Geometry: see drawing. Coordinates: mm, zero at the bounding-box minimum. A direction names the side the tool comes from. Give positions to 0.01 mm unless a question says otherwise; leave off trailing zeros. Write each loop counter-clockwise with the first axis right and the second up, starting at its lowest first coordinate (ties: lowest second). Pieces come first, ordered by that corner, then holes. Notation, with made-up numbers: (48.5, -25) -> (79.5, -25) arc R30 cw to (79.5, 9) -> close; hole circle Ø8 at (7.5, 77). An arc over 180 degrees is marked (long way). Use one line per item in the form item = value. Start each with the question number.
(1) Set-up query: the marked faces 3 and 4. Return all of +Z, -Z, +X, -X, +Y, -Y with unobstructed straight access to the full face (end or side cutting, diameter ignored); none if empty.
(2) Material intervals for line 1 along X through (y, z) = (8.75, 14); line 2 along X through (y, z) = (9.25, 41); line 3 along Z through (x, y) = (35.5, 12), sorted ascending. Write a range as from..to.
(3) First-contact query: P1, Ø2, axis at x = 26, z = 26, coming from the -Y side; P2, Ø11.5, axis at x = 29.5, z = 32.5, coming from the +Y side. Flat tips, straight axial feed; report the tip coordinate or a pass-through.
(4) Cut plane A-A, the plane z = 33. Output: boundary loops of the cut face in (x, y).
(5) Cut plane D-D, the plane x = 71.5. Output: boundary loops of the cut face in (y, z).
(6) Cut plane C-C, the plane z = 21.5. Output: boundary loops of the cut face in (x, y), and give its area (3 significant figures).
(7) Draft query along X for the marked faces 1 and 2. Return one class per face: pulls with the +X half, pulls with the -X half, needs draft (parallel to the pull), parting line crosses it, or undercut.
(8) Cut plane B-B, the plane x = 170.5. Output: boundary loops of the cut face in (y, z).
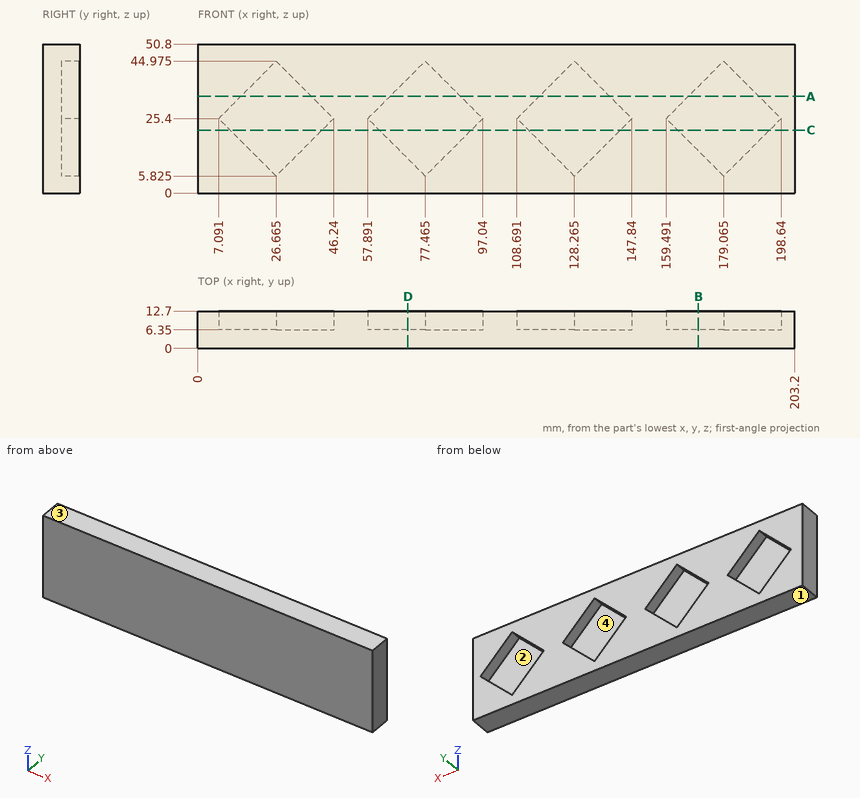
Geometry says:
q1.face_3 = +Z, +X, -X, +Y, -Y
q1.face_4 = +Y
q2.line_1 = 0..18.49, 34.84..69.29, 85.64..120.09, 136.44..170.89, 187.24..203.2
q2.line_2 = 0..22.69, 30.64..73.49, 81.44..124.29, 132.24..175.09, 183.04..203.2
q2.line_3 = 0..14.66, 36.14..50.8
q3.P1 = 0
q3.P2 = 6.35
q4.outline = (0, 0) -> (203.2, 0) -> (203.2, 12.7) -> (191.04, 12.7) -> (191.04, 6.35) -> (167.09, 6.35) -> (167.09, 12.7) -> (140.24, 12.7) -> (140.24, 6.35) -> (116.29, 6.35) -> (116.29, 12.7) -> (89.44, 12.7) -> (89.44, 6.35) -> (65.49, 6.35) -> (65.49, 12.7) -> (38.64, 12.7) -> (38.64, 6.35) -> (14.69, 6.35) -> (14.69, 12.7) -> (0, 12.7) -> close
q5.outline = (0, 0) -> (12.7, 0) -> (12.7, 11.79) -> (6.35, 11.79) -> (6.35, 39.01) -> (12.7, 39.01) -> (12.7, 50.8) -> (0, 50.8) -> close
q6.outline = (0, 0) -> (203.2, 0) -> (203.2, 12.7) -> (194.74, 12.7) -> (194.74, 6.35) -> (163.39, 6.35) -> (163.39, 12.7) -> (143.94, 12.7) -> (143.94, 6.35) -> (112.59, 6.35) -> (112.59, 12.7) -> (93.14, 12.7) -> (93.14, 6.35) -> (61.79, 6.35) -> (61.79, 12.7) -> (42.34, 12.7) -> (42.34, 6.35) -> (10.99, 6.35) -> (10.99, 12.7) -> (0, 12.7) -> close
q6.area = 1,780 mm^2
q7.face_1 = needs draft
q7.face_2 = undercut
q8.outline = (0, 0) -> (12.7, 0) -> (12.7, 14.39) -> (6.35, 14.39) -> (6.35, 36.41) -> (12.7, 36.41) -> (12.7, 50.8) -> (0, 50.8) -> close
